The listing builds one solid part. Answer for the finished solid, in the listing's coordinates (mm). A direction names the side the tool comes from. Give positions to 0.01 mm unless a question says otherwise; leave off trailing zeros. Order: outer loops, then holes, each group sorted by start corner. A loop starts at its lowest first (then second) coordinate and runs counter-clockwise, first axis right, second up. Notation, with made-up numbers: (60.5, 37.25) -> (114.5, 37.25) arc R7 ccw to (114.5, 48.25) -> close; hole circle Ø3 at (43.25, 76.25). An arc over 180 degrees is marked (long way). Answer as a JSON object with one key per item and string values. Group by question number.
```python
from build123d import *
from OCP.BRepFilletAPI import BRepFilletAPI_MakeChamfer

# Parameters (mm, degrees)
SKETCH1_W                                            = 390.7
SKETCH1_H                                            = 132.7
MAINBODY_DEPTH                                       = 18.5
SKETCH2_W                                            = 390.7
SKETCH2_H                                            = 132.7
SKETCH2_W_2                                          = 386.7
SKETCH2_H_2                                          = 128.7
ALIGMENTLIP_DEPTH                                    = 2
TYPINGANGLE_DEPTH                                    = 414.035143783
SKETCH4_W                                            = 372
SKETCH4_H                                            = 122
PCBCUTOUT_DEPTH                                      = 3
M2_CLEARANCE_HOLE2_D                                 = 2.4
CUT_EXTRUDE2_START                                   = -1
SKETCH11_R                                           = 2.5
CUT_EXTRUDE2_DEPTH                                   = 412.911649145
SKETCH12_W                                           = 15
SKETCH12_H                                           = 2.5
CUT_EXTRUDE3_DEPTH                                   = 3
FILLET1_R                                            = 2.5
SKETCH13_W                                           = 15
SKETCH13_H                                           = 20
CUT_EXTRUDE4_DEPTH                                   = 2
FILLET2_R                                            = 4
CUT_EXTRUDE7_START                                   = -11.833363055
CUT_EXTRUDE7_OUTLINE_W                               = 2
CUT_EXTRUDE7_OUTLINE_H                               = 17.5
CUT_EXTRUDE7_OUTLINE_H_2                             = 7.5
CUT_EXTRUDE7_OUTLINE_H_3                             = 10
CUT_EXTRUDE7_OUTLINE_R                               = 1
CUT_EXTRUDE7_DEPTH                                   = 11.833363055
FILLET3_R                                            = 1
CHAMFER1_SIZE                                        = 0.5
CHAMFER1_SIZE2                                       = 0.561801899
CUT_EXTRUDE10_START                                  = -2.5
SKETCH18_R                                           = 20
SKETCH18_W                                           = 25
SKETCH18_H                                           = 28
CUT_EXTRUDE10_DEPTH                                  = 410.891093571
FILLET4_R                                            = 1
CSK_FOR_M3_FLAT_HEAD_MACHINE_SCREW1_D                = 3.4
CSK_FOR_M3_FLAT_HEAD_MACHINE_SCREW1_CSINK_D          = 6.37874
CSK_FOR_M3_FLAT_HEAD_MACHINE_SCREW1_CSINK_ANGLE      = 90
CSK_FOR_M3_FLAT_HEAD_MACHINE_SCREW1_ON_F_D           = 3.4
CSK_FOR_M3_FLAT_HEAD_MACHINE_SCREW1_ON_F_CSINK_D     = 6.37874
CSK_FOR_M3_FLAT_HEAD_MACHINE_SCREW1_ON_F_CSINK_ANGLE = 90


# Read off the part's stored shape, not the designer's step: Cut-Extrude7
with BuildPart() as part:
    # Sketch1 → MainBody (new body)
    with BuildSketch(Plane(origin=(0, 0, 0), x_dir=(1, 0, 0), z_dir=(0, 1, 0))):
        with Locations((195.35, 66.35)):
            Rectangle(SKETCH1_W, SKETCH1_H)
    extrude(amount=MAINBODY_DEPTH)

    # Sketch2 → AligmentLip (cut)
    with BuildSketch(Plane(origin=(0, 18.5, 0), x_dir=(1, 0, 0), z_dir=(0, 1, 0))):
        with Locations((195.35, 66.35)):
            Rectangle(SKETCH2_W, SKETCH2_H)
        with Locations((195.35, 66.35)):
            Rectangle(SKETCH2_W_2, SKETCH2_H_2, mode=Mode.SUBTRACT)
    extrude(amount=-ALIGMENTLIP_DEPTH, mode=Mode.SUBTRACT)

    # Sketch3 → TypingAngle (cut, through all)
    with BuildSketch(Plane.ZY):
        Polygon((-116.028888387, 0), (-132.7, 13.5), (-132.7, 0), align=None)
        Polygon((0, 12.195127583), (-116.028888387, 0), (0, 0), align=None)
    extrude(amount=-TYPINGANGLE_DEPTH, mode=Mode.SUBTRACT)

    # Sketch4 → PCBCutout (cut)
    with BuildSketch(Plane(origin=(0, 18.5, 0), x_dir=(1, 0, 0), z_dir=(0, 1, 0))):
        with Locations((195.35, 66.35)):
            Rectangle(SKETCH4_W, SKETCH4_H)
    extrude(amount=-PCBCUTOUT_DEPTH, mode=Mode.SUBTRACT)

    # M2 Clearance Hole2 (through all)
    with Locations(Plane(origin=(110, 18.5, -129), x_dir=(0, 0, 1), z_dir=(0, 1, 0))):
        with Locations((0, 0), (17.65, -104.3), (62.65, -104.3), (107.65, -104.3), (125.3, 0), (0, 170.7), (125.3, 170.7), (107.65, 275), (62.65, 275), (17.65, 275)):
            Hole(M2_CLEARANCE_HOLE2_D / 2)

    # Sketch11 → Cut-Extrude2 (cut, through all)
    with BuildSketch(Plane(origin=(0, 15.5, 0), x_dir=(1, 0, 0), z_dir=(0, 1, 0)).offset(CUT_EXTRUDE2_START)):
        with Locations(Location((110, 129, 0), (0, 0, 270))):
            Circle(SKETCH11_R)
        with Locations(Location((5.7, 111.35, 0), (0, 0, 270))):
            Circle(SKETCH11_R)
        with Locations(Location((5.7, 66.35, 0), (0, 0, 270))):
            Circle(SKETCH11_R)
        with Locations(Location((5.7, 21.35, 0), (0, 0, 270))):
            Circle(SKETCH11_R)
        with Locations(Location((110, 3.7, 0), (0, 0, 270))):
            Circle(SKETCH11_R)
        with Locations(Location((280.7, 3.7, 0), (0, 0, 270))):
            Circle(SKETCH11_R)
        with Locations(Location((385, 21.35, 0), (0, 0, 270))):
            Circle(SKETCH11_R)
        with Locations(Location((385, 66.35, 0), (0, 0, 270))):
            Circle(SKETCH11_R)
        with Locations(Location((385, 111.35, 0), (0, 0, 270))):
            Circle(SKETCH11_R)
        with Locations(Location((280.7, 129, 0), (0, 0, 90))):
            Circle(SKETCH11_R)
    extrude(amount=-CUT_EXTRUDE2_DEPTH, mode=Mode.SUBTRACT)

    # Sketch12 → Cut-Extrude3 (cut)
    with BuildSketch(Plane(origin=(0, 18.5, 0), x_dir=(1, 0, 0), z_dir=(0, 1, 0))):
        with Locations((35.9, 128.6)):
            Rectangle(SKETCH12_W, SKETCH12_H)
    extrude(amount=-CUT_EXTRUDE3_DEPTH, mode=Mode.SUBTRACT)

    # Fillet1
    fillet1_edges = [part.edges().sort_by_distance(p)[0] for p in [
        (43.4, 17, -129.85),
        (28.4, 17, -129.85),
    ]]
    fillet(fillet1_edges, radius=FILLET1_R - 0.0001)  # a hair under: the kernel refuses the full size

    # Sketch13 → Cut-Extrude4 (cut)
    with BuildSketch(Plane(origin=(0, 15.5, 0), x_dir=(1, 0, 0), z_dir=(0, 1, 0))):
        with Locations((16.85, 66.35)):
            Rectangle(SKETCH13_W, SKETCH13_H)
    extrude(amount=-CUT_EXTRUDE4_DEPTH, mode=Mode.SUBTRACT)

    # Fillet2
    fillet2_edges = [part.edges().sort_by_distance(p)[0] for p in [
        (388.7, 17.5, -130.7),
        (2, 17.5, -130.7),
        (2, 17.5, -2),
        (388.7, 17.5, -2),
        (9.35, 14.5, -56.35),
        (9.35, 14.5, -76.35),
        (24.35, 14.5, -76.35),
        (24.35, 14.5, -56.35),
        (9.35, 17, -5.35),
        (9.35, 17, -127.35),
        (381.35, 17, -127.35),
        (381.35, 17, -5.35),
    ]]
    fillet(fillet2_edges, radius=FILLET2_R)

    # Cut-Extrude7 outline → Cut-Extrude7 (cut)
    with BuildSketch(Plane(origin=(0, 12.061881184, -1.267754798), x_dir=(1, 0, 0), z_dir=(0, -0.9945218953682734, 0.10452846326765429)).offset(CUT_EXTRUDE7_START)):
        with Locations((202.1, -60.945229197)):
            Rectangle(CUT_EXTRUDE7_OUTLINE_W, CUT_EXTRUDE7_OUTLINE_H)
        with BuildLine():
            Line((196.6, -79.695229197), (198.6, -79.695229197))
            Line((198.6, -79.695229197), (198.6, -59.695229197))
            Line((198.6, -59.695229197), (196.6, -59.695229197))
            Line((196.6, -59.695229197), (196.6, -72.204912456))
            Line((196.6, -72.204912456), (193.1, -72.21107453))
            ThreePointArc((193.1, -72.21107453), (192.115845333, -73.195229197), (193.1, -74.179383864))
            Line((193.1, -74.179383864), (196.6, -74.185545938))
            Line((196.6, -74.185545938), (196.6, -79.695229197))
        make_face()
        with Locations((207.1, -55.445229197)):
            Rectangle(CUT_EXTRUDE7_OUTLINE_W, CUT_EXTRUDE7_OUTLINE_H_2)
        with Locations((184.1, -65.195229197)):
            Rectangle(CUT_EXTRUDE7_OUTLINE_W, CUT_EXTRUDE7_OUTLINE_H_3)
        with Locations((188.6, -65.195229197)):
            Rectangle(CUT_EXTRUDE7_OUTLINE_W, CUT_EXTRUDE7_OUTLINE_H_3)
        with Locations((193.1, -65.195229197)):
            Rectangle(CUT_EXTRUDE7_OUTLINE_W, CUT_EXTRUDE7_OUTLINE_H_3)
        with Locations((202.1, -73.195229197)):
            Circle(CUT_EXTRUDE7_OUTLINE_R)
    extrude(amount=CUT_EXTRUDE7_DEPTH, mode=Mode.SUBTRACT)

    # Fillet3
    fillet3_edges = [part.edges().sort_by_distance(p)[0] for p in [
        (183.1, 10.63488319, -61.644572613),
        (187.6, 10.63488319, -61.644572613),
        (192.1, 10.63488319, -61.644572613),
        (185.1, 10.63488319, -61.644572613),
        (189.6, 10.63488319, -61.644572613),
        (194.1, 10.63488319, -61.644572613),
        (185.1, 10.112240874, -71.644723487),
        (189.6, 10.112240874, -71.644723487),
        (194.1, 10.112240874, -71.644723487),
        (183.1, 10.112240874, -71.644723487),
        (187.6, 10.112240874, -71.644723487),
        (192.1, 10.112240874, -71.644723487),
        (196.6, 9.615730673, -81.144866818),
        (198.6, 9.615730673, -81.144866818),
        (196.6, 10.661015306, -61.144565069),
        (198.6, 10.661015306, -61.144565069),
        (201.1, 11.052997043, -53.644451913),
        (203.1, 11.052997043, -53.644451913),
        (206.1, 11.079129159, -53.144444369),
        (208.1, 11.079129159, -53.144444369),
        (208.1, 10.687147422, -60.644557525),
        (206.1, 10.687147422, -60.644557525),
        (201.1, 10.13837299, -71.144715944),
        (203.1, 10.13837299, -71.144715944),
    ]]
    fillet(fillet3_edges, radius=FILLET3_R - 0.0001)  # a hair under: the kernel refuses the full size

    # Chamfer1: one chamfer whose edges measure the first distance from different faces: ONE call of the kernel's chamfer builder (chamfer() names one face for all edges)
    chamfer1_edges_1 = [part.edges().sort_by_distance(p)[0] for p in [
        (0, 15, -132.7),
        (390.7, 15, -132.7),
        (390.7, 14.347563791, 0),
        (0, 14.347563791, 0),
        (195.35, 16.5, -132.7),
        (390.7, 16.5, -66.35),
        (195.35, 16.5, 0),
        (0, 16.5, -66.35),
        (0, 6.75, -124.364444193),
        (390.7, 6.75, -124.364444193),
        (0, 6.097563791, -58.014444193),
        (390.7, 6.097563791, -58.014444193),
    ]]
    chamfer1_edges_2 = [part.edges().sort_by_distance(p)[0] for p in [
        (195.35, 12.195127583, 0),
    ]]
    chamfer1_side_2 = [part.faces().sort_by_distance(p)[0] for p in [
        (195.35, 14.347563791, 0),
    ]]
    chamfer1 = BRepFilletAPI_MakeChamfer(part.part.solid().wrapped)
    for e in chamfer1_edges_1:
        chamfer1.Add(CHAMFER1_SIZE, e.wrapped)
    for e in chamfer1_edges_2:
        chamfer1.Add(CHAMFER1_SIZE, CHAMFER1_SIZE2, e.wrapped, chamfer1_side_2[0].wrapped)  # the first distance lies on this face
    add(Compound.cast(chamfer1.Shape()), mode=Mode.REPLACE)

    # Sketch18 → Cut-Extrude10 (cut, through all)
    # profile 1 of 3: a face of its own
    with BuildSketch(Plane(origin=(0, 12.061881184, -1.267754798), x_dir=(1, 0, 0), z_dir=(0, -0.9945218953682734, 0.10452846326765429)).offset(CUT_EXTRUDE10_START)):
        with Locations(Location((195.6, -65.695229197, 0), (0, 0, 270))):
            Circle(SKETCH18_R)
        with Locations((195.6, -65.695229197)):
            Rectangle(SKETCH18_W, SKETCH18_H, mode=Mode.SUBTRACT)
    # profile 2 of 3: a face of its own
    with BuildSketch(Plane(origin=(0, 12.061881184, -1.267754798), x_dir=(1, 0, 0), z_dir=(0, -0.9945218953682734, 0.10452846326765429)).offset(CUT_EXTRUDE10_START)):
        Polygon((183.1, -51.695229197), (208.1, -79.695229197), (183.1, -79.695229197), align=None)
    # profile 3 of 3: a face of its own
    with BuildSketch(Plane(origin=(0, 12.061881184, -1.267754798), x_dir=(1, 0, 0), z_dir=(0, -0.9945218953682734, 0.10452846326765429)).offset(CUT_EXTRUDE10_START)):
        Polygon((208.1, -51.695229197), (183.1, -51.695229197), (208.1, -79.695229197), align=None)
    extrude(amount=-CUT_EXTRUDE10_DEPTH, mode=Mode.SUBTRACT)

    # Fillet4
    fillet4_edges = [part.edges().sort_by_distance(p)[0] for p in [
        (196.6, 5.757565014, -73.207781767),
        (196.6, 5.55053244, -75.177565132),
    ]]
    fillet(fillet4_edges, radius=FILLET4_R)

    # CSK for M3 Flat Head Machine Screw1 (through all)
    with Locations(Plane(origin=(213.1, 5.194859832, -66.603098655), x_dir=(0, -0.104528463268, -0.994521895368), z_dir=(0, -0.994521895368, 0.104528463268))):
        with Locations((0, 0)):
            CounterSinkHole(CSK_FOR_M3_FLAT_HEAD_MACHINE_SCREW1_D / 2, CSK_FOR_M3_FLAT_HEAD_MACHINE_SCREW1_CSINK_D / 2, counter_sink_angle=CSK_FOR_M3_FLAT_HEAD_MACHINE_SCREW1_CSINK_ANGLE)

    # CSK for M3 Flat Head Machine Screw1 on f (through all)
    with Locations(Plane(origin=(178.1, 5.194859832, -66.603098655), x_dir=(0, -0.104527994185, -0.994521944671), z_dir=(0, -0.994521944671, 0.104527994185))):
        with Locations((0, 0)):
            CounterSinkHole(CSK_FOR_M3_FLAT_HEAD_MACHINE_SCREW1_ON_F_D / 2, CSK_FOR_M3_FLAT_HEAD_MACHINE_SCREW1_ON_F_CSINK_D / 2, counter_sink_angle=CSK_FOR_M3_FLAT_HEAD_MACHINE_SCREW1_ON_F_CSINK_ANGLE)


solid = part.part
```
(1) Which of the six approach directions +Z, -Z, +X, -X, +Y, -Y give full straight-line access (tool end or side, diameter ignored) to faces 4 (the flat face through (17, 13.5, -66)), 5 (the flat face through (137, 18.5, -5))?
(2) A cutting plane is placed at A-A (x = 249.5). Determine the outline of the cut face in (y, z).
(3) For a pull along X with two mould halves and no side action, classify faces 1 (the flat face through (390.45, 6.85, -124.09)), 2 (the flat face through (195.32, 7.71, -66.59)), 3 (the flat face through (192.622, 6.656, -124.248)) as +X half, -X half, draft (parallel to the pull), parting line (faces both ways), or undercut.
(4) A cutting plane is placed at B-B (z = -97). Determine the outline of the cut face in (x, y).
(5) Find the intervals of material crossed by line 1 along X through (y, z) = (1.5, -111); line 2 along X through (y, z) = (17.05, -21.35); line 3 along Z through (x, y) = (385, 15.75), in increasing order. Write a range as [from, to].
(6) Flat-ended cylindrical pins translate along their axes: pin 1 Ø3 at (x, z) = (280.7, -129) entering from +Y; pin 2 Ø4 at (x, z) = (6.5, -21.5) entering from -Y; pin 3 Ø2 at (x, z) = (264.5, -39.5) entering from +Y; pin 4 Ø2 at (x, z) = (5.7, -21.35) entering from +Y. Find the tip coordinate at first contact, or state that the pin passes through.
Check sheet entries:
{
 "1": {"face 4": "+Y", "face 5": "+Z, -Z, +X, -X, +Y"},
 "2": {"outline": "(0, -116.03) -> (13.5, -132.7) -> (16, -132.7) -> (16.5, -132.2) -> (16.5, -130.7) -> (18.5, -130.7) -> (18.5, -127.35) -> (15.5, -127.35) -> (15.5, -5.35) -> (18.5, -5.35) -> (18.5, -2) -> (16.5, -2) -> (16.5, -0.5) -> (16, 0) -> (12.7, 0) -> (12.14, -0.56) -> close"},
 "3": {"face 1": "+X half", "face 2": "undercut", "face 3": "draft"},
 "4": {"outline": "(0, 2.5) -> (0.5, 2) -> (390.2, 2) -> (390.7, 2.5) -> (390.7, 16) -> (390.2, 16.5) -> (388.7, 16.5) -> (388.7, 18.5) -> (381.35, 18.5) -> (381.35, 15.5) -> (9.35, 15.5) -> (9.35, 18.5) -> (2, 18.5) -> (2, 16.5) -> (0.5, 16.5) -> (0, 16) -> close"},
 "5": {"line 1": "x = [0, 3.22], [8.18, 382.52], [387.48, 390.7]", "line 2": "x = [2, 4.5], [6.9, 9.35], [381.35, 383.8], [386.2, 388.7]", "line 3": "z = [-132.7, -112.55], [-110.15, -67.55], [-65.15, -22.55], [-20.15, 0]"},
 "6": {"pin 1": "stops at y = 18.5", "pin 2": "stops at y = 9.74", "pin 3": "stops at y = 15.5", "pin 4": "passes through"}
}
